from build123d import *

# Parameters (mm, degrees)
F0_R      = 101.6
F1_DEPTH  = 12.7
F1_FACE_R = 101.6
F2_DEPTH  = 50.8
F2_TAPER  = 25
F3_R      = 6.35


with BuildPart() as f1:
    # F0 (on Top) → F1 (new body)
    with BuildSketch(Plane.XY):
        Circle(F0_R)
    extrude(amount=F1_DEPTH)

    # F1_face (on face) → F2 (join)
    with BuildSketch(Plane.XY.offset(12.7)):
        Circle(F1_FACE_R)
    extrude(amount=F2_DEPTH, taper=F2_TAPER)

    # F3
    f3_edges = [f1.edges().sort_by_distance(p)[0] for p in [
        (-101.6, 0, 12.7),
    ]]
    fillet(f3_edges, radius=F3_R)


solid = f1.part
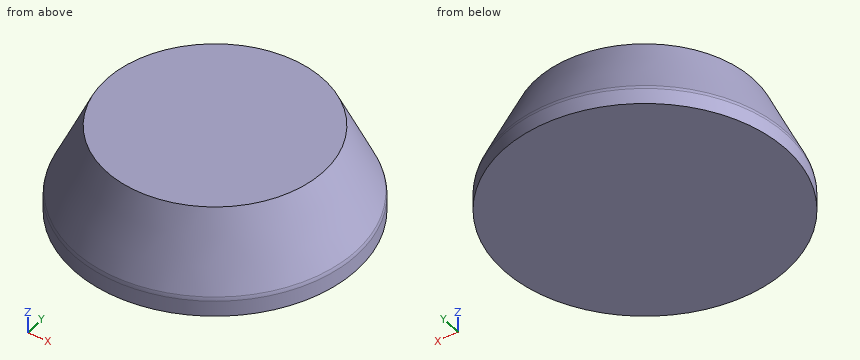
The listing builds one solid part. Answer for the finished solid, in the listing's coordinates (mm). Coordinates: 2 decimals unless noted, no trailing zeros. Order: outer loops, then holes, each group sorted by start corner. A loop starts at its lowest first (then second) coordinate and runs counter-clockwise, first axis right, second up. Notation, with made-up numbers: M 22.25,5.5 L 55.25,5.5 A20 cw 55.25,10.5 Z; hole C -25,59.25 d3. An arc over 180 degrees is marked long. Use CSV: the item, a comma, the result in double quotes.
Q1. Given pin 1 Ø2 at (y, z) = (-7.5, 21) entering from -X; pin 2 Ø2 at (y, z) = (10, 7) entering from -X; pin 3 Ø1 at (x, z) = (-74.5, 48.5) entering from -Y, each flat-ended and moving along its own axis, determine where each tip first touches the part or whether it passes through.
Here are the results:
pin 1,"x = -97.92"
pin 2,"x = -101.2"
pin 3,"y = -41.75"
Q2. Straight lines are drawn through the part: L1, parallel to Y at x = -78, z = 26; L2, parallel to Y at x = -7.5, z = 61; L3, parallel to Z at x = 78, y = -35. For each, find the intervals that lie inside material, in ascending order.
Here are the results:
L1,"-54.93 to 54.93"
L2,"-78.72 to 78.72"
L3,"0 to 47.24"
Q3. Section B-B (z = 46) is taken. Determine the outline of the cut face in (x, y).
Here are the results:
outline,"C 0,0 d172.14"
Q4. Section A-A (z = 8) is taken. Determine the outline of the cut face in (x, y).
Here are the results:
outline,"C 0,0 d203.2"
